For this review, use the dimensioned drawing (mm, ordinates from the lowest corner) and the shaded views. A direction names the side the tool comes from. Coordinates: 2 decimals unless noted, no trailing zeros. Loops run counter-clockwise (first coordinate to the right, second up) from the corner with the lowest first, then second, coordinate; pieces in that order, holes last. Notation, with made-up numbers: (-32, 65.25) - (6, 65.25) arc R8 ccw to (6, 70.25) - close; hole circle Ø11 at (-23, 55). An arc over 180 degrees is marked (long way). Answer in a Markdown table with one row per item. Add a question column.
(1) Mouldability with a two-part tool opening along Z and no side actions: class the marked faces 3, 4 and 5 as +Z half, -Z half, draft (parallel to the pull), parting line (faces both ways), or undercut.
(2) For P1, Ø1.5, axis at x = 4, y = 17, coming from the +Z side; P2, Ø2, axis at x = 6, y = 9, coming from the +Z side (1 decimal); P3, Ø1.5, axis at x = 6.5, z = 4.5, coming from the -Y side (1 decimal), all flat-tipped, find the tip position at first contact; note any pin that passes through.
(3) Machinability: for the marked faces 1 and 2, which of the approach directions +Z, -Z, +X, -X, +Y, -Y give a long, thin tool a straight path to every point of the face, cutting with its end or side? Answer none if there is none.
(4) For line 1 along Y through (x, z) = (5.75, 12.7); line 2 along X through (y, z) = (2, 12.5); line 3 along Y through (x, z) = (8.5, 12.7), list the stretches that pass through material, from the lowest coordinate up.
(5) We need section A-A on z = 12.7. Write out the cut boundary in (x, y), plus the area to 3 significant figures.
(6) We need section C-C on x = 8.5. Write out the cut boundary in (y, z), plus the area to 3 significant figures.
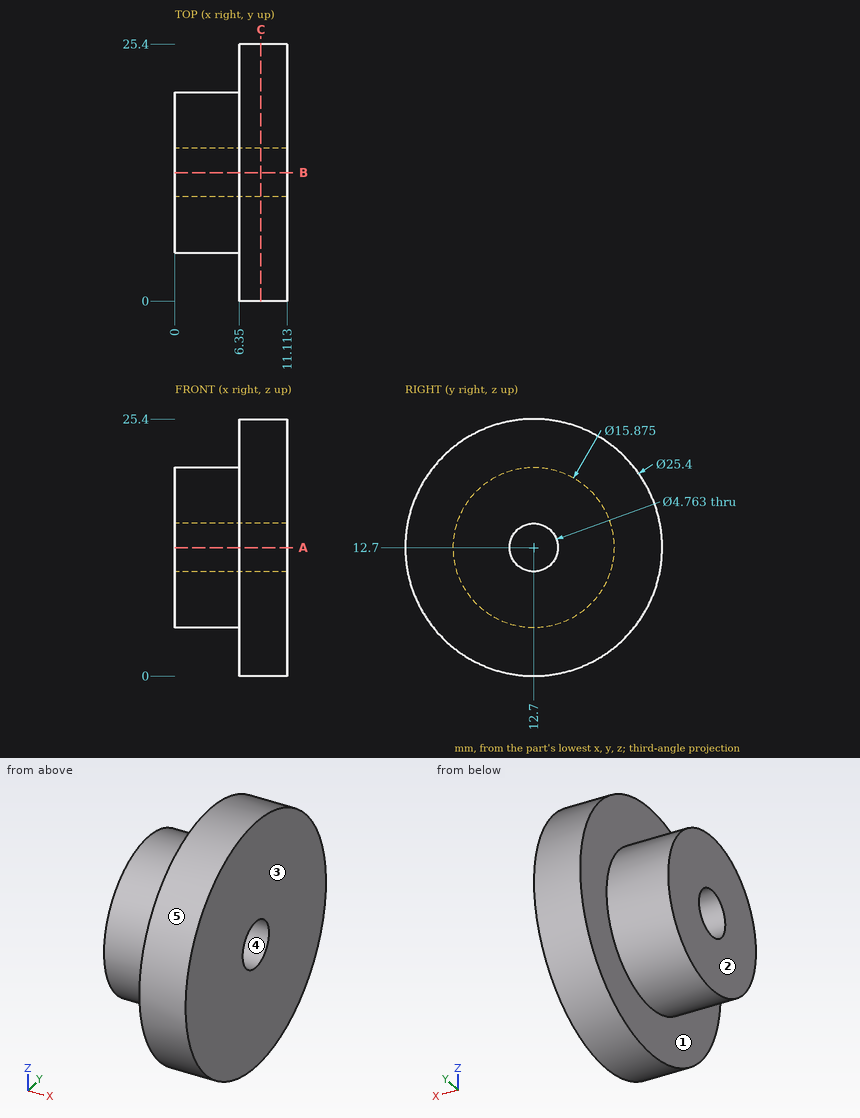
Outcome:
| question | item | result |
|---|---|---|
| 1 | face 3 | draft |
| 1 | face 4 | undercut |
| 1 | face 5 | parting line |
| 2 | P1 | z = 19.8 |
| 2 | P2 | z = 25.1 |
| 2 | P3 | y = 2.4 |
| 3 | face 1 | -X |
| 3 | face 2 | +Z, -Z, -X, +Y, -Y |
| 4 | line 1 | 4.76 to 10.32, 15.08 to 20.64 |
| 4 | line 2 | 6.35 to 11.11 |
| 4 | line 3 | 0 to 10.32, 15.08 to 25.4 |
| 5 | outline | (0, 4.76) - (6.35, 4.76) - (6.35, 0) - (11.11, 0) - (11.11, 10.32) - (0, 10.32) - close; (0, 15.08) - (11.11, 15.08) - (11.11, 25.4) - (6.35, 25.4) - (6.35, 20.64) - (0, 20.64) - close |
| 5 | area | 169 mm² |
| 6 | outline | circle Ø25.4 at (12.7, 12.7); hole circle Ø4.76 at (12.7, 12.7) |
| 6 | area | 489 mm² |
